The listing builds one solid part. Answer for the finished solid, in the listing's coordinates (mm). A direction names the side the tool comes from. Coordinates: 2 decimals unless noted, no trailing zeros. Loops run counter-clockwise (first coordinate to the right, second up) from the corner with the lowest first, then second, coordinate; pieces in that order, holes last. Notation, with made-up numbers: M -17,-11.5 L 36,-11.5 A31 cw 36,21.5 Z; hole C 34,1.5 d6. An arc over 180 degrees is marked long. Answer in a Markdown table with one row per item. Add a question column.
from build123d import *

# Parameters (mm, degrees)
EXTRUDE_1_DEPTH     = 4
FILLET_1_R          = 2
CUT_EXTRUDE_1_REACH = 33.064
SKETCH_3_R          = 2.75
EXTRUDE_2_DEPTH     = 2


with BuildPart() as part:
    # 草图1 → 凸台-拉伸1 (new body)
    with BuildSketch(Plane(origin=(0, 0, 0), x_dir=(1, 0, 0), z_dir=(0, 1, 0))):
        Polygon((-25, 13), (25, 13), (25, -13), (10, -13), (10, -18), (-10, -18), (-10, -13), (-25, -13), align=None)
    extrude(amount=EXTRUDE_1_DEPTH)

    # 圆角1
    fillet_1_edges = [part.edges().sort_by_distance(p)[0] for p in [
        (10, 2, 18),
        (-10, 2, 18),
        (-25, 2, 13),
        (-25, 2, -13),
        (25, 2, -13),
        (25, 2, 13),
    ]]
    fillet(fillet_1_edges, radius=FILLET_1_R)

    # 草图3 → 切除-拉伸1 (cut, up to next)
    with BuildSketch(Plane(origin=(0, 4, 0), x_dir=(1, 0, 0), z_dir=(0, 1, 0)), mode=Mode.PRIVATE) as cut_extrude_1_sk1:
        with Locations(Location((-15, 0, 0), (0, 0, 270))):
            Circle(SKETCH_3_R)
    cut_extrude_1_tool1 = extrude(cut_extrude_1_sk1.sketch, amount=-CUT_EXTRUDE_1_REACH, mode=Mode.PRIVATE) & part.part
    # 草图3 → 切除-拉伸1 (cut, up to next)
    with BuildSketch(Plane(origin=(0, 4, 0), x_dir=(1, 0, 0), z_dir=(0, 1, 0)), mode=Mode.PRIVATE) as cut_extrude_1_sk2:
        with Locations(Location((15, 0, 0), (0, 0, 90))):
            Circle(SKETCH_3_R)
    cut_extrude_1_tool2 = extrude(cut_extrude_1_sk2.sketch, amount=-CUT_EXTRUDE_1_REACH, mode=Mode.PRIVATE) & part.part
    add(cut_extrude_1_tool1.solids().sort_by_distance((-15, 4, 0))[0], mode=Mode.SUBTRACT)
    add(cut_extrude_1_tool2.solids().sort_by_distance((15, 4, 0))[0], mode=Mode.SUBTRACT)

    # 草图4 → 凸台-拉伸2 (add)
    with BuildSketch(Plane(origin=(0, 4, 0), x_dir=(1, 0, 0), z_dir=(0, 1, 0))):
        Polygon((21, -9.5), (21, 9.5), (21, 10), (-8.5, 10), (-20.5, 10), (-21, 10), (-21, 9.5), (-21, -9.5), (-23, -9.5), (-23, 11), (23, 11), (23, -9.5), align=None)
    extrude(amount=EXTRUDE_2_DEPTH)


solid = part.part
(1) Each of these flat-tipped pins is pushed along its axis until it touches: pin 1 (1.6 mm diameter, centred on x = -21.5, y = 5, fed in from +Z); pin 2 (1.2 mm diameter, centred on x = -16, y = 1.5, fed in from +Z); pin 3 (1.5 mm diameter, centred on y = 3, z = 14, fed in from +X). Where does it stop, or does it pass through?
(2) Straight lines are drawn through the part: line 1 (X direction, y = 3.05, z = 0); line 2 (Z direction, x = 15, y = 2.1); line 3 (X direction, y = 5, z = 8). For each, find the intervals that lie inside material, in ascending order.
(3) The mould has two halves that part along X. Classify faces 1 (the face through (-12.273, 2.028, -0.358)), 2 (the face through (-16, 2, 13)), 3 (the face through (9.43, 2.03, 17.4)), 4 (the face through (-9.4, 2.03, 17.43)): released by +X, released by -X, zero draft, split by the parting line, or undercut.
(4) For faces 5 (the face through (0, 5, -10)), 6 (the face through (0, 5, -11)), 7 (the face through (22, 5, 9.5)), 8 (the face through (17, 2, 13)), determine the directions among +Z, -Z, +X, -X, +Y, -Y from which every point of the face is accessible in a straight line to the end or side of a thin tool.
(5) A cutting plane is placed at D-D (z = 5.5). Give the vertices of the cut face in (x, y).
(6) A cutting plane is placed at B-B (y = 1.9). Give the vertices of the cut face in (x, z).
(7) A cutting plane is placed at C-C (x = -15). Give the vertices of the cut face in (y, z), plus the area to 3 significant figures.
(8) A cutting plane is placed at A-A (z = 0). Give the vertices of the cut face in (x, y), plus the area to 3 significant figures.
Solved:
| question | item | result |
|---|---|---|
| 1 | pin 1 | stops at z = 9.5 |
| 1 | pin 2 | stops at z = 13 |
| 1 | pin 3 | stops at x = 10 |
| 2 | line 1 | x = -25 to -17.75, -12.25 to 12.25, 17.75 to 25 |
| 2 | line 2 | z = -13 to -2.75, 2.75 to 13 |
| 2 | line 3 | x = -23 to -21, 21 to 23 |
| 3 | face 1 | undercut |
| 3 | face 2 | zero draft |
| 3 | face 3 | released by +X |
| 3 | face 4 | released by -X |
| 4 | face 5 | +Z, +Y |
| 4 | face 6 | -Z, +X, -X, +Y |
| 4 | face 7 | +Z, +X, -X, +Y |
| 4 | face 8 | +Z, +X, +Y, -Y |
| 5 | outline | M -25,0 L 25,0 L 25,4 L 23,4 L 23,6 L 21,6 L 21,4 L -21,4 L -21,6 L -23,6 L -23,4 L -25,4 Z |
| 6 | outline | M -25,-11 A2 ccw -23,-13 L 23,-13 A2 ccw 25,-11 L 25,11 A2 ccw 23,13 L 10,13 L 10,16 A2 ccw 8,18 L -8,18 A2 ccw -10,16 L -10,13 L -23,13 A2 ccw -25,11 Z; hole C -15,0 d5.5; hole C 15,0 d5.5 |
| 7 | outline | M 0,-13 L 4,-13 L 4,-11 L 6,-11 L 6,-10 L 4,-10 L 4,-2.75 L 0,-2.75 Z; M 0,2.75 L 4,2.75 L 4,13 L 0,13 Z |
| 7 | area | 84.0 mm² |
| 8 | outline | M -25,0 L -17.75,0 L -17.75,4 L -21,4 L -21,6 L -23,6 L -23,4 L -25,4 Z; M -12.25,0 L 12.25,0 L 12.25,4 L -12.25,4 Z; M 17.75,0 L 25,0 L 25,4 L 23,4 L 23,6 L 21,6 L 21,4 L 17.75,4 Z |
| 8 | area | 164 mm² |
